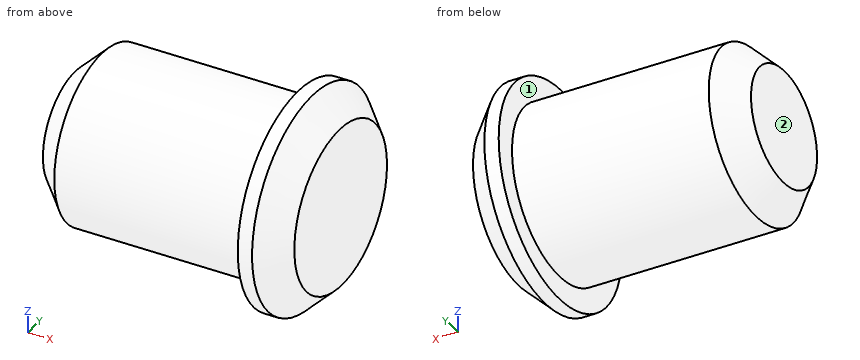
```python
from build123d import *

# Parameters (mm, degrees)
F0_W    = 19.05
F0_H    = 7.1755
F2_SIZE = 2.286


with BuildPart() as f1:
    # F0 (on Top) → F1 (revolve)
    with BuildSketch(Plane.XY):
        with Locations((0, 3.58775)):
            Rectangle(F0_W, F0_H)
        Polygon((9.525, 7.1755), (9.525, 0), (13.0302, 0), (13.0302, 9.144), (9.525, 9.144), align=None)
    revolve(axis=Axis((6.400125, 0, 0), (1, 0, 0)))

    # F2
    f2_edges = [f1.edges().sort_by_distance(p)[0] for p in [
        (13.0302, -9.144, 0),
        (-9.525, -7.1755, 0),
    ]]
    chamfer(f2_edges, length=F2_SIZE)


solid = f1.part
```
Read the model definition and answer for the solid it produces. Units are mm, in the model's axes. Face numbers are marked on the shaded views. A direction names the side the tool comes from. Give positions to 0.01 mm unless a question says otherwise; leave off trailing zeros. Write each loop counter-clockwise with the first axis right and the second up, starting at its lowest first coordinate (ties: lowest second). Pieces come first, ordered by that corner, then holes. Notation, with made-up numbers: (-9.5, 88.5) -> (30.5, 88.5) arc R26 cw to (30.5, 126.5) -> close; hole circle Ø1 at (0.25, 0.25). An arc over 180 degrees is marked (long way). Answer in a Markdown table with one row per item.
1) Section A-A on y = 0 is taken. Give the vertices of the cut face in (x, z) (1 decimal), plus the area to 3 significant figures.
Results list:
| item | result |
|---|---|
| outline | (-9.5, -4.9) -> (-7.2, -7.2) -> (9.5, -7.2) -> (9.5, -9.1) -> (10.7, -9.1) -> (13, -6.9) -> (13, 6.9) -> (10.7, 9.1) -> (9.5, 9.1) -> (9.5, 7.2) -> (-7.2, 7.2) -> (-9.5, 4.9) -> close |
| area | 327 mm^2 |
2) Each of these flat-tipped pins is pushed along its axis until it touches: pin 1 Ø8 at (x, y) = (-4, 0.5) entering from +Z; pin 2 Ø6 at (x, z) = (3.5, -6) entering from -Y; pin 3 Ø6 at (x, z) = (7.5, 2.5) entering from +Y. Where does it stop, or does it pass through?
Results list:
| item | result |
|---|---|
| pin 1 | z = 7.18 |
| pin 2 | y = -6.52 |
| pin 3 | y = 9.14 |
3) A tool of negligible diameter and unlimited length cuts with its end or side. For the marked faces 1 and 2, from which of +Z, -Z, +X, -X, +Y, -Y can it reach the whole face along a straight path? Write none if from no direction.
Results list:
| item | result |
|---|---|
| face 1 | -X |
| face 2 | +Z, -Z, -X, +Y, -Y |
4) Section D-D on x = 11.25 is taken. Give the vertices of the cut face in (y, z).
Results list:
| item | result |
|---|---|
| outline | circle Ø17.28 at (0, 0) |
5) Section C-C on x = -6.75 is taken. Give the vertices of the cut face in (y, z).
Results list:
| item | result |
|---|---|
| outline | circle Ø14.35 at (0, 0) |
6) Straight lines are drawn through the part: line 1 (Z direction, x = -0.5, y = 0); line 2 (Y direction, x = 10.5, z = 2.5); line 3 (Y direction, x = 1.75, z = 3). For each, find the intervals that lie inside material, in ascending order. Write a range as [from, to].
Results list:
| item | result |
|---|---|
| line 1 | [-7.18, 7.18] |
| line 2 | [-8.8, 8.8] |
| line 3 | [-6.52, 6.52] |
